Here's how the part is built. I have some questions about the finished solid (model axes, mm). A direction names the side the tool comes from. Round coordinates to 2 decimals unless told otherwise and drop trailing zeros. Write each loop counter-clockwise with the first axis right and the second up, starting at its lowest first coordinate (ties: lowest second). Pieces come first, ordered by that corner, then holes. Notation, with made-up numbers: (5, 10.5) - (12, 10.5) arc R22 ccw to (12, 20.5) - close; hole circle Ø5 at (-8.75, 65). An arc over 180 degrees is marked (long way). Return JSON: item names as keys, results as strings. Group by question number.
Autodesk Inventor part; units mm, degrees
ref_plane "YZ Plane" through (0, 0, 0) normal (1, 0, 0) x (0, 1, 0)
ref_plane "XZ Plane" through (0, 0, 0) normal (0, 1, 0) x (-1, 0, 0)
ref_plane "XY Plane" through (0, 0, 0) normal (0, 0, 1) x (1, 0, 0)
sketch "Sketch1" plane through (0, 0, 0) normal (0, 0, 1) x (1, 0, 0)
  line L0 (-50, -69) -> (50, -69)
  line L1 (50, -69) -> (50, 69)
  line L2 (50, 69) -> (-50, 69)
  line L3 (-50, 69) -> (-50, -69)
  line L4 (-50, -69) -> (50, 69) construction
  line L5 (50, -69) -> (-50, 69) construction
  line L6 (30, -49) -> (-30, -49)
  line L7 (-30, -49) -> (-30, 49)
  line L8 (-30, 49) -> (30, 49)
  line L9 (30, 49) -> (30, -49)
  line L10 (30, -49) -> (-30, 49) construction
  line L11 (-30, -49) -> (30, 49) construction
  point P0 (0, 0)
  dimension "d172" = 60
  dimension "d180" = 20
  dimension "d181" = 20
  dimension "d182" = 98
extrude "Plate5" add sketch "Sketch1" along normal blind 3
sketch "Sketch9" plane through (0, 0, 3) normal (0, 0, 1) x (1, 0, 0)
  circle A0 centre (43, -62) radius 3
  line L0 (43, 62) -> (-43, 62) construction
  line L1 (-43, 62) -> (-43, -62) construction
  line L2 (-43, -62) -> (43, -62) construction
  line L3 (43, -62) -> (43, 62) construction
  line L4 (43, 62) -> (-43, -62) construction
  line L5 (-43, 62) -> (43, -62) construction
  circle A1 centre (-43, -62) radius 3
  circle A2 centre (43, 62) radius 3
  circle A3 centre (-43, 62) radius 3
  line L6 (-30, -49) -> (-30, 49)
  line L7 (-30, 49) -> (30, 49)
  line L8 (30, 49) -> (30, -49)
  line L9 (30, -49) -> (-30, -49)
  line L10 (50, -69) -> (-50, -69)
  line L11 (50, 69) -> (50, -69)
  line L12 (-50, 69) -> (50, 69)
  line L13 (-50, -69) -> (-50, 69)
  circle A4 centre (-43, 0) radius 3 construction
  circle A5 centre (43, 0) radius 3 construction
  point P0 (0, 0)
  dimension "d174" = 6
  dimension "d183" = 7
  dimension "d184" = 7
extrude "Cut2" cut sketch "Sketch9" against normal blind 3 contours A0 | A1 | A2 | A3
fillet "Corner Round1" radius 6 4 edges at (50, 69, 1.5) (-50, 69, 1.5) (-50, -69, 1.5) (50, -69, 1.5)
properties part number "PRS 940-51 FDS Diam way flange 1" material "Stainless Steel"
1) If we mould it in two halves opening along X, with no side actions, what happens to faces 3 (the flat face through (-34, 1, 0)), 4 (the flat face through (50, -1, 1)), 5 (the cylindrical face through (40.79, -59.97, 1.52)), 6 (the flat face through (-50, 1, 1))? For each: released by +X, released by -X, zero draft, split by the parting line, or undercut.
2) Imagine slicing it at B-B (x = 21). Please give me the cut outline in (y, z).
3) Will this pin go through, and if not, where does the flat tip stop? pin 1 Ø7 at (x, y) = (-43, -62) entering from +Z.
4) For faces 1 (the flat face through (0, -49, 1)), 2 (the cylindrical face through (-48.289, -67.196, 1.521)), which set-ups out of +Z, -Z, +X, -X, +Y, -Y let a thin tool reach every point of the face, with its end or its side?
5) Imagine slicing it at A-A (y = -27). Please give me the cut outline in (x, z).
6) I need wall thicknesses on line 1 along Y through (x, z) = (-43, 2.3); line 2 along Y through (x, z) = (-6.5, 1.3); line 3 along X through (y, z) = (-18.5, 1.85). Which ranges of each line are inside material? Lowest first, please.
7) Imagine slicing it at C-C (z = 0.75). Please give me the cut outline in (x, y), plus the area to 3 significant figures.
Results found:
{
 "1": {"face 3": "zero draft", "face 4": "released by +X", "face 5": "undercut", "face 6": "released by -X"},
 "2": {"outline": "(-69, 0) - (-49, 0) - (-49, 3) - (-69, 3) - close; (49, 0) - (69, 0) - (69, 3) - (49, 3) - close"},
 "3": {"pin 1": "stops at z = 3"},
 "4": {"face 1": "+Z, -Z", "face 2": "+Z, -Z, -X, -Y"},
 "5": {"outline": "(-50, 0) - (-30, 0) - (-30, 3) - (-50, 3) - close; (30, 0) - (50, 0) - (50, 3) - (30, 3) - close"},
 "6": {"line 1": "y = -69 to -65, -59 to 59, 65 to 69", "line 2": "y = -69 to -49, 49 to 69", "line 3": "x = -50 to -30, 30 to 50"},
 "7": {"outline": "(-50, -63) arc R6 ccw to (-44, -69) - (44, -69) arc R6 ccw to (50, -63) - (50, 63) arc R6 ccw to (44, 69) - (-44, 69) arc R6 ccw to (-50, 63) - close; hole circle Ø6 at (-43, -62); hole circle Ø6 at (-43, 62); hole (-30, -49) - (30, -49) - (30, 49) - (-30, 49) - close; hole circle Ø6 at (43, -62); hole circle Ø6 at (43, 62)", "area": "7,780 mm²"}
}
